```python
from build123d import *

# Parameters (mm, degrees)
BOSS_EXTRUDE2_DEPTH      = 2
CUT_EXTRUDE2_DEPTH       = 7
SKETCH10_W               = 40
SKETCH10_H               = 1
BOSS_EXTRUDE3_DEPTH      = 7
CUT_EXTRUDE4_DEPTH       = 1
CUT_EXTRUDE5_DEPTH       = 1
SKETCH14_R               = 1.75
BOSS_EXTRUDE4_DEPTH      = 6.600028
SKETCH15_R               = 2.75
BOSS_EXTRUDE5_DEPTH      = 5
BOSS_EXTRUDE7_DEPTH      = 2
BOSS_EXTRUDE7_DEPTH_BACK = 2
BOSS_EXTRUDE8_DEPTH      = 3
SKETCH21_R               = 3
CUT_EXTRUDE7_DEPTH       = 1.9
SKETCH22_R               = 1.4
CUT_EXTRUDE8_DEPTH       = 15


with BuildPart() as part:
    # Sketch3 → Boss-Extrude2 (new body)
    with BuildSketch(Plane(origin=(0, 0, 0), x_dir=(1, 0, 0), z_dir=(0, 1, 0))):
        with BuildLine():
            Line((-30.001043465, -34.015189653), (57.998956535, -34.015189653))
            ThreePointArc((57.998956535, -34.015189653), (65.070024347, -31.086257464), (67.998956535, -24.015189653))
            Line((67.998956535, -24.015189653), (67.998956535, 40.984810347))
            ThreePointArc((67.998956535, 40.984810347), (65.070024347, 48.055878159), (57.998956535, 50.984810347))
            Line((57.998956535, 50.984810347), (-30.001043465, 50.984810347))
            ThreePointArc((-30.001043465, 50.984810347), (-37.072111277, 48.055878159), (-40.001043465, 40.984810347))
            Line((-40.001043465, 40.984810347), (-40.001043465, -24.015189653))
            ThreePointArc((-40.001043465, -24.015189653), (-37.072111277, -31.086257464), (-30.001043465, -34.015189653))
        make_face()
    extrude(amount=BOSS_EXTRUDE2_DEPTH)

    # Sketch6 → Cut-Extrude2 (cut)
    with BuildSketch(Plane(origin=(0, 2, 0), x_dir=(1, 0, 0), z_dir=(0, 1, 0))):
        with BuildLine():
            Line((-18.182060551, 10.483778137), (-20.721753803, 10.483778137))
            ThreePointArc((-20.721753803, 10.483778137), (-22.720721593, 8.484810347), (-20.721753803, 6.485842558))
            Line((-20.721753803, 6.485842558), (-18.182060551, 6.485842558))
            ThreePointArc((-18.182060551, 6.485842558), (-11.809060764, 8.484810347), (-18.182060551, 10.483778137))
        make_face()
    extrude(amount=-CUT_EXTRUDE2_DEPTH, mode=Mode.SUBTRACT)

    # Sketch10 → Boss-Extrude3 (add)
    with BuildSketch(Plane(origin=(0, 0, 0), x_dir=(1, 0, 0), z_dir=(0, 1, 0))):
        with Locations((39.263184903, 46.984810347)):
            Rectangle(SKETCH10_W, SKETCH10_H)
        with Locations((39.263184903, -30.015189653)):
            Rectangle(SKETCH10_W, SKETCH10_H)
    extrude(amount=BOSS_EXTRUDE3_DEPTH)

    # Sketch12 → Cut-Extrude4 (cut)
    with BuildSketch(Plane.XY.offset(30.515189653)):
        with BuildLine():
            Line((56.263184903, 7), (59.263184903, 7))
            Line((59.263184903, 7), (59.263184903, 4))
            ThreePointArc((59.263184903, 4), (58.384505246, 6.121320344), (56.263184903, 7))
        make_face()
        with BuildLine():
            Line((19.263184903, 4), (19.263184903, 7))
            Line((19.263184903, 7), (22.263184903, 7))
            ThreePointArc((22.263184903, 7), (20.141864559, 6.121320344), (19.263184903, 4))
        make_face()
    extrude(amount=-CUT_EXTRUDE4_DEPTH, mode=Mode.SUBTRACT)

    # Sketch13 → Cut-Extrude5 (cut)
    with BuildSketch(Plane(origin=(0, 0, -47.484810347), x_dir=(-1, 0, 0), z_dir=(0, 0, -1))):
        with BuildLine():
            Line((-56.263184903, 7), (-59.263184903, 7))
            Line((-59.263184903, 7), (-59.263184903, 4))
            ThreePointArc((-59.263184903, 4), (-58.384505246, 6.121320344), (-56.263184903, 7))
        make_face()
        with BuildLine():
            Line((-19.263184903, 4), (-19.263184903, 7))
            Line((-19.263184903, 7), (-22.263184903, 7))
            ThreePointArc((-22.263184903, 7), (-20.141864559, 6.121320344), (-19.263184903, 4))
        make_face()
    extrude(amount=-CUT_EXTRUDE5_DEPTH, mode=Mode.SUBTRACT)

    # Sketch14 → Boss-Extrude4 (add)
    with BuildSketch(Plane.XZ):
        with Locations((-29.011006112, 25.011760646)):
            Circle(SKETCH14_R)
        with Locations((14.981881874, 25.011760646)):
            Circle(SKETCH14_R)
        with Locations((14.981881874, -40.988239354)):
            Circle(SKETCH14_R)
        with Locations((-29.011006112, -40.988239354)):
            Circle(SKETCH14_R)
    extrude(amount=-BOSS_EXTRUDE4_DEPTH)

    # Sketch15 → Boss-Extrude5 (add)
    with BuildSketch(Plane.XZ):
        with Locations((-29.011006112, 25.011760646)):
            Circle(SKETCH15_R)
        with Locations((14.981881874, 25.011760646)):
            Circle(SKETCH15_R)
        with Locations((14.981881874, -40.988239354)):
            Circle(SKETCH15_R)
        with Locations((-29.011006112, -40.988239354)):
            Circle(SKETCH15_R)
    extrude(amount=-BOSS_EXTRUDE5_DEPTH)

    # Sketch19 → Boss-Extrude7 (add, two sides)
    with BuildSketch(Plane(origin=(-7, 0, 0), x_dir=(0, 0, -1), z_dir=(1, 0, 0))) as boss_extrude7_sk:
        with BuildLine():
            add(Edge.make_bspline(
                [(45.56151484, 5.184913415), (45.252793653, 7.279810059), (43.062728824, 7.229305282)],
                knots=[0, 0, 0, 1, 1, 1], degree=2))
            Line((43.062728824, 7.229305282), (46.416379445, 10.690814493))
            Line((46.416379445, 10.690814493), (47.06151484, 10.690814493))
            Line((47.06151484, 10.690814493), (47.06151484, 2.75))
            ThreePointArc((47.06151484, 2.75), (46.841844926, 2.219669914), (46.31151484, 2))
            Line((46.31151484, 2), (46.31151484, 0))
            Line((46.31151484, 0), (44.81151484, 0))
            Line((44.81151484, 0), (44.81151484, 2))
            ThreePointArc((44.81151484, 2), (45.341844926, 2.219669914), (45.56151484, 2.75))
            Line((45.56151484, 2.75), (45.56151484, 5.184913415))
        make_face()
        with BuildLine():
            Line((-29.44675875, 10.690814493), (-30.091894145, 10.690814493))
            Line((-30.091894145, 10.690814493), (-30.091894145, 2.75))
            ThreePointArc((-30.091894145, 2.75), (-29.872224231, 2.219669914), (-29.341894145, 2))
            Line((-29.341894145, 2), (-29.341894145, 0))
            Line((-29.341894145, 0), (-28.591894145, 0))
            Line((-28.591894145, 0), (-27.841894145, 0))
            Line((-27.841894145, 0), (-27.841894145, 2))
            ThreePointArc((-27.841894145, 2), (-28.372224231, 2.219669914), (-28.591894145, 2.75))
            Line((-28.591894145, 2.75), (-28.591894145, 5.184913415))
            add(Edge.make_bspline(
                [(-28.591894145, 5.184913415), (-28.283172958, 7.279810059), (-26.09310813, 7.229305282)],
                knots=[0, 0, 0, 1, 1, 1], degree=2))
            Line((-26.09310813, 7.229305282), (-29.44675875, 10.690814493))
        make_face()
    extrude(amount=BOSS_EXTRUDE7_DEPTH)
    extrude(boss_extrude7_sk.sketch, amount=-BOSS_EXTRUDE7_DEPTH_BACK)

    # Sketch5 → Boss-Extrude8 (add)
    with BuildSketch(Plane(origin=(0, 0, 34.015189653), x_dir=(1, 0, 0), z_dir=(0, 1, 0))):
        with BuildLine():
            Line((-36.001043465, 78.5), (-39.368540462, 78.5))
            ThreePointArc((-39.368540462, 78.5), (-39.841647358, 76.778346145), (-40.001043465, 75))
            Line((-40.001043465, 75), (-40.001043465, 72.5))
            Line((-40.001043465, 72.5), (-36.001043465, 72.5))
            ThreePointArc((-36.001043465, 72.5), (-33.001043465, 75.5), (-36.001043465, 78.5))
        make_face()
        with BuildLine():
            Line((63.998956535, 78.5), (67.366453533, 78.5))
            ThreePointArc((67.366453533, 78.5), (67.839560429, 76.778346145), (67.998956535, 75))
            Line((67.998956535, 75), (67.998956535, 72.5))
            Line((67.998956535, 72.5), (63.998956535, 72.5))
            ThreePointArc((63.998956535, 72.5), (60.998956535, 75.5), (63.998956535, 78.5))
        make_face()
        with BuildLine():
            Line((63.998956535, 12.5), (67.998956535, 12.5))
            Line((67.998956535, 12.5), (67.998956535, 10))
            ThreePointArc((67.998956535, 10), (67.839560429, 8.221653855), (67.366453533, 6.5))
            Line((67.366453533, 6.5), (63.998956535, 6.5))
            ThreePointArc((63.998956535, 6.5), (60.998956535, 9.5), (63.998956535, 12.5))
        make_face()
        with BuildLine():
            Line((-36.001043465, 12.5), (-40.001043465, 12.5))
            Line((-40.001043465, 12.5), (-40.001043465, 10))
            ThreePointArc((-40.001043465, 10), (-39.841647358, 8.221653855), (-39.368540462, 6.5))
            Line((-39.368540462, 6.5), (-36.001043465, 6.5))
            ThreePointArc((-36.001043465, 6.5), (-33.001043465, 9.5), (-36.001043465, 12.5))
        make_face()
    extrude(amount=BOSS_EXTRUDE8_DEPTH)

    # Sketch21 → Cut-Extrude7 (cut)
    with BuildSketch(Plane.XZ):
        with Locations((-36.001043465, 24.515189653)):
            Circle(SKETCH21_R)
        with Locations((63.998956535, 24.515189653)):
            Circle(SKETCH21_R)
        with Locations((63.998956535, -41.484810347)):
            Circle(SKETCH21_R)
        with Locations((-36.001043465, -41.484810347)):
            Circle(SKETCH21_R)
    extrude(amount=-CUT_EXTRUDE7_DEPTH, mode=Mode.SUBTRACT)

    # Sketch22 → Cut-Extrude8 (cut)
    with BuildSketch(Plane.XZ.offset(-1.9)):
        with Locations((-36.001043465, 24.515189653)):
            Circle(SKETCH22_R)
        with Locations((63.998956535, 24.515189653)):
            Circle(SKETCH22_R)
        with Locations((63.998956535, -41.484810347)):
            Circle(SKETCH22_R)
        with Locations((-36.001043465, -41.484810347)):
            Circle(SKETCH22_R)
    extrude(amount=-CUT_EXTRUDE8_DEPTH, mode=Mode.SUBTRACT)


solid = part.part
```
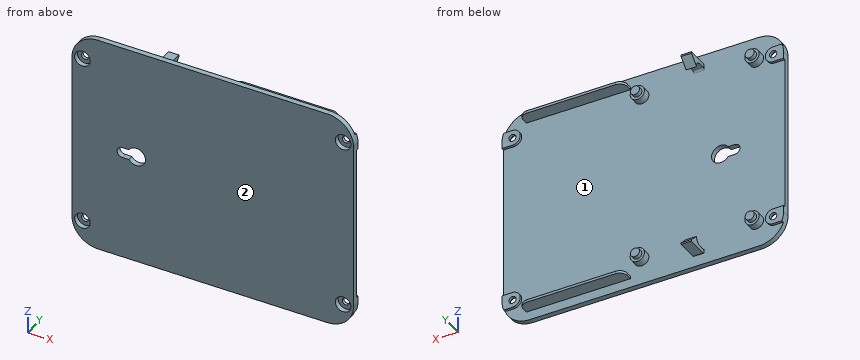
Model file for the job. Use its own axes, mm. Face numbers are marked on the shaded views. Coordinates: 2 decimals unless noted, no trailing zeros. Order: outer loops, then holes, each group sorted by start corner. A loop starts at its lowest first (then second) coordinate and runs counter-clockwise, first axis right, second up. Notation, with made-up numbers: (31, 52.5) -> (54, 52.5) arc R33 cw to (54, 81.5) -> close; hole circle Ø5 at (34, -37.5). An arc over 180 degrees is marked (long way). Return JSON: item names as keys, results as strings.
Item 1: Slice it at C-C (z = -28). Write the cut outline in (x, y), then the cut area to 3 significant figures.
Model answer:
{"outline": "(-40, 0) -> (68, 0) -> (68, 2) -> (-40, 2) -> close", "area": "216 mm²"}
Item 2: Mould opens along Z. For the marked faces 1 and 2 say: pulls with the +Z half, pulls with the -Z half, needs draft (parallel to the pull), parting line crosses it, or undercut.
Model answer:
{"face 1": "undercut", "face 2": "needs draft"}
Item 3: Pin check, flat tips, straight feed: P1, Ø6.5, axis at x = -35, z = 25, coming from the -Y side; P2, Ø0.8, axis at y = 3, z = -47, coming from the -X side; P3, Ø0.5, axis at y = 3.5, z = 30, coming from the +X side; P4, Ø8, axis at x = 43.5, z = -29.5, coming from the +Y side. Stop position of each tip, or through.
Model answer:
{"P1": "stops at y = 0", "P2": "stops at x = -9", "P3": "stops at x = 59.26", "P4": "stops at y = 2"}
Item 4: Slice it at D-D (x = 8.5). Write the cut outline in (y, z), then the cut area to 3 significant figures.
Model answer:
{"outline": "(0, -50.98) -> (2, -50.98) -> (2, 34.02) -> (0, 34.02) -> close", "area": "170 mm²"}
Item 5: Slice it at B-B (z = -8). Write the cut outline in (x, y).
Model answer:
{"outline": "(-40, 0) -> (-22.66, 0) -> (-22.66, 2) -> (-40, 2) -> close; (-11.84, 0) -> (68, 0) -> (68, 2) -> (-11.84, 2) -> close"}
Item 6: Wall check: line 1 along Z through (x, y) = (38.5, 4.5); line 2 along Y through (x, z) = (55.5, -20.5); line 3 along X through (y, z) = (6.5, 24). Give the ranges that are in metal, low to high. Write a range as from..to.
Model answer:
{"line 1": "z = -47.48..-46.48, 29.52..30.52", "line 2": "y = 0..2", "line 3": "x = -30.44..-27.58, 13.55..16.41"}
Item 7: Slice it at A-A (x = 53). Write the cut outline in (y, z).
Model answer:
{"outline": "(0, -50.98) -> (2, -50.98) -> (2, -47.48) -> (7, -47.48) -> (7, -46.48) -> (2, -46.48) -> (2, 29.52) -> (7, 29.52) -> (7, 30.52) -> (2, 30.52) -> (2, 34.02) -> (0, 34.02) -> close"}
